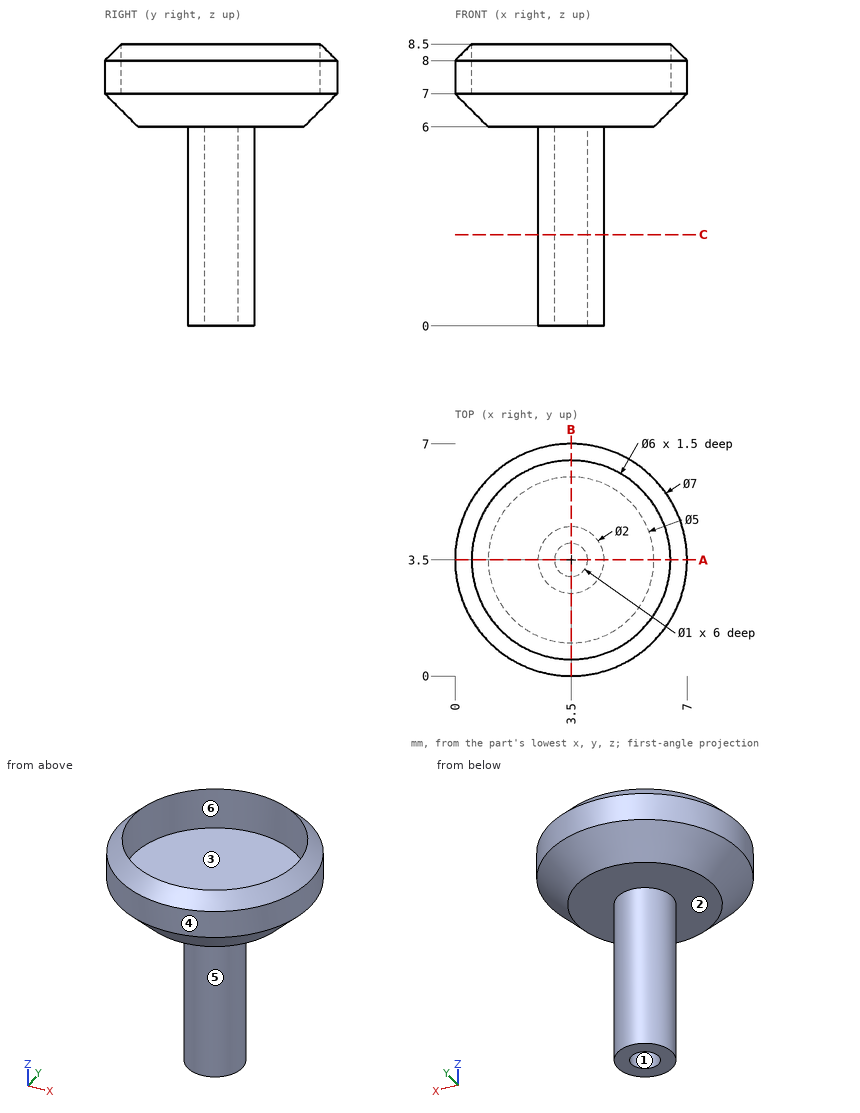
The drawing under review shows one solid part. Ordinate dimensions are in mm from its lowest x, y, z. A direction names the side the tool comes from. Coordinates: 2 decimals unless noted, no trailing zeros. Write each loop counter-clockwise with the first axis right and the second up, starting at its lowest first coordinate (ties: lowest second). Pieces come first, ordered by that corner, then holes. Notation, with made-up numbers: M 74,-11 L 90,-11 A11 cw 90,5 Z; hole C -29.75,29 d4. An arc over 180 degrees is marked long. Put each result on its own line as item: value.
1) Draft analysis for pull direction Y (two halves, no side actions). For the marked faces 1, 2, 3 and 4, state which applies: released by +Y, released by -Y, zero draft, split by the parting line, or undercut.
Computed:
face 1: undercut
face 2: zero draft
face 3: undercut
face 4: split by the parting line
2) Add section A-A on y = 3.5. Give the boundary of the cut face in (x, z).
Computed:
outline: M 0,7 L 1,6 L 2.5,6 L 2.5,0 L 3,0 L 3,6 L 4,6 L 4,0 L 4.5,0 L 4.5,6 L 6,6 L 7,7 L 7,8 L 6.5,8.5 L 6.5,7 L 0.5,7 L 0.5,8.5 L 0,8 Z
3) Clearance check with flat-ended pins moving along their axes: pin 1 Ø4 at (x, z) = (2, 1) entering from -Y; pin 2 Ø1.8 at (x, y) = (2.5, 3.5) entering from +Z; pin 3 Ø0.8 at (x, y) = (3.5, 3.5) entering from -Z. State where each tip first meets the part, or that it passes through.
Computed:
pin 1: stops at y = 2.5
pin 2: stops at z = 7
pin 3: stops at z = 6
4) For the marked faces 5 and 6, list the 3-axis set-ups (+Z, -Z, +X, -X, +Y, -Y) from which the entire face can be reached by the end or side of a thin tool; tool diameter is ignored.
Computed:
face 5: -Z
face 6: +Z
5) Wall thickness on probe 1 along Y at (x, z) = (3.5, 7.45); probe 2 along Y at (x, z) = (3.5, 3.1); probe 3 along Z at (x, y) = (5.5, 4.5): over which ranges is each line inside the solid? List them lowest first. Write a range as [from, to].
Computed:
probe 1: y = [0, 0.5], [6.5, 7]
probe 2: y = [2.5, 3], [4, 4.5]
probe 3: z = [6, 7]
6) Add section C-C on z = 2.75. Give the boundary of the cut face in (x, y).
Computed:
outline: C 3.5,3.5 d2; hole C 3.5,3.5 d1
